from build123d import *

# Parameters (mm, degrees)
F1_DEPTH = 15.24


# Not quite as in the source:
# - a feature names something its author has since deleted; it is built from what else it names


with BuildPart() as f1:
    # F0 (on Top) → F1 (new body)
    with BuildSketch(Plane.XY):
        with BuildLine():
            ThreePointArc((-6.8469626463, 19.8860116913), (-11.313708499, 23.0332541473), (-14.4609509549, 27.5))
            Line((-14.4609509549, 27.5), (-27.5, 14.4609509549))
            Line((-27.5, 14.4609509549), (-21.1890490451, 8.15))
            Line((-21.1890490451, 8.15), (-13.0390490451, 0))
            Line((-13.0390490451, 0), (0, 13.0390490451))
            Line((0, 13.0390490451), (-6.8469626463, 19.8860116913))
        make_face()
        Polygon((-13.0390490451, 0), (-21.1890490451, 8.15), (-21.1890490451, -8.15), align=None)
        with BuildLine():
            Line((14.4609509549, -27.5), (27.5, -14.4609509549))
            Line((27.5, -14.4609509549), (21.1890490451, -8.15))
            Line((21.1890490451, -8.15), (13.0390490451, 0))
            Line((13.0390490451, 0), (0, -13.0390490451))
            Line((0, -13.0390490451), (6.8469626463, -19.8860116913))
            ThreePointArc((6.8469626463, -19.8860116913), (11.313708499, -23.0332541473), (14.4609509549, -27.5))
        make_face()
        Polygon((13.0390490451, 0), (0, 13.0390490451), (0, 0), (0, -13.0390490451), align=None)
        Polygon((0, 0), (0, 13.0390490451), (-13.0390490451, 0), (0, -13.0390490451), align=None)
        with BuildLine():
            Line((27.5, 14.4609509549), (14.4609509549, 27.5))
            ThreePointArc((14.4609509549, 27.5), (11.313708499, 23.0332541473), (6.8469626463, 19.8860116913))
            Line((6.8469626463, 19.8860116913), (0, 13.0390490451))
            Line((0, 13.0390490451), (13.0390490451, 0))
            Line((13.0390490451, 0), (21.1890490451, 8.15))
            Line((21.1890490451, 8.15), (27.5, 14.4609509549))
        make_face()
        Polygon((21.1890490451, -8.15), (21.1890490451, 8.15), (13.0390490451, 0), align=None)
        with BuildLine():
            Line((0, -13.0390490451), (-6.8469626463, -19.8860116913))
            ThreePointArc((-6.8469626463, -19.8860116913), (-3.5089018739, -18.7364659329), (0, -18.3469626463))
            Line((0, -18.3469626463), (0, -13.0390490451))
        make_face()
        with BuildLine():
            Line((0, 13.0390490451), (6.8469626463, 19.8860116913))
            ThreePointArc((6.8469626463, 19.8860116913), (3.5089018739, 18.7364659329), (0, 18.3469626463))
            Line((0, 18.3469626463), (0, 13.0390490451))
        make_face()
        with BuildLine():
            ThreePointArc((0, 18.3469626463), (-3.5089018739, 18.7364659329), (-6.8469626463, 19.8860116913))
            Line((-6.8469626463, 19.8860116913), (0, 13.0390490451))
            Line((0, 13.0390490451), (0, 18.3469626463))
        make_face()
        with BuildLine():
            Line((6.8469626463, -19.8860116913), (0, -13.0390490451))
            Line((0, -13.0390490451), (0, -18.3469626463))
            ThreePointArc((0, -18.3469626463), (3.5089018739, -18.7364659329), (6.8469626463, -19.8860116913))
        make_face()
        with BuildLine():
            Line((-21.1890490451, -8.15), (-27.5, -14.4609509549))
            Line((-27.5, -14.4609509549), (-14.4609509549, -27.5))
            ThreePointArc((-14.4609509549, -27.5), (-11.313708499, -23.0332541473), (-6.8469626463, -19.8860116913))
            Line((-6.8469626463, -19.8860116913), (0, -13.0390490451))
            Line((0, -13.0390490451), (-13.0390490451, 0))
            Line((-13.0390490451, 0), (-21.1890490451, -8.15))
        make_face()
    extrude(amount=F1_DEPTH)


solid = f1.part
Check sheet for the modelled part. Datum: model origin and axes. Units: mm. A direction names the side the tool comes from. Round coordinates to 2 decimals unless told otherwise and drop trailing zeros. Loops run counter-clockwise (first coordinate to the right, second up) from the corner with the lowest first, then second, coordinate; pieces in that order, holes last.
1. Sectioned sample at B-B on z = 8. Record the boundary of the cut face in (x, y), and give its area (3 significant figures).
2. Scan lines: probe 1 along X at (y, z) = (-7, 10.25); probe 2 along X at (y, z) = (-23.5, 9.25); probe 3 along Y at (x, z) = (22.5, 8). Record each from-to range of solid material in increasing order.
3. Sectioned sample at D-D on x = 10. Record the boundary of the cut face in (y, z).
4. Sectioned sample at A-A on x = 22.5. Record the boundary of the cut face in (y, z).
5. Mould release check, pull along Y, two halves, no side actions. Record for faces 1 (the flat face through (24.39, -11.35, 7.51)), 2 (the flat face through (20.89, -21.07, 7.51)), 3 (the flat face through (-24.39, 11.35, 7.51)), 4 (the flat face through (21.07, 20.89, 7.51)): released by +Y, released by -Y, zero draft, split by the parting line, or undercut.
6. Gauge pin test, flat ends, axial feed: pin 1 Ø5 at (y, z) = (-10, 6.5) entering from +X; pin 2 Ø5 at (y, z) = (8.5, 12) entering from -X; pin 3 Ø8 at (y, z) = (-7, 5) entering from +X; pin 4 Ø6 at (x, z) = (15.5, 9.5) entering from -Y. Record the tip position at first contact, or that the pin passes through.
7. Sectioned sample at C-C on y = -4.5. Record the boundary of the cut face in (x, z), and give its area (3 significant figures).
8. Set-up check for faces 5 (the flat face through (21.189, 0, 8)), 6 (the flat face through (-21.07, -20.89, 7.51)), 7 (the flat face through (-24.3, -11.26, 7.51)): record each of +Z, -Z, +X, -X, +Y, -Y from which the full face is reachable in a straight line by a thin tool's end or side.
Recorded:
1. outline: (-27.5, -14.46) - (-14.46, -27.5) arc R16 cw to (14.46, -27.5) - (27.5, -14.46) - (21.19, -8.15) - (21.19, 8.15) - (27.5, 14.46) - (14.46, 27.5) arc R16 cw to (-14.46, 27.5) - (-27.5, 14.46) - (-21.19, 8.15) - (-21.19, -8.15) - close
1. area: 2,020 mm2
2. probe 1: x = -21.19 to 21.19
2. probe 2: x = -18.46 to -11.76, 11.76 to 18.46
2. probe 3: y = -19.46 to -9.46, 9.46 to 19.46
3. outline: (-21.86, 0) - (21.86, 0) - (21.86, 15.24) - (-21.86, 15.24) - close
4. outline: (-19.46, 0) - (-9.46, 0) - (-9.46, 15.24) - (-19.46, 15.24) - close; (9.46, 0) - (19.46, 0) - (19.46, 15.24) - (9.46, 15.24) - close
5. face 1: undercut
5. face 2: released by -Y
5. face 3: undercut
5. face 4: released by +Y
6. pin 1: stops at x = 25.54
6. pin 2: stops at x = -24.04
6. pin 3: stops at x = 24.04
6. pin 4: stops at y = -27.5
7. outline: (-21.19, 0) - (21.19, 0) - (21.19, 15.24) - (-21.19, 15.24) - close
7. area: 646 mm2
8. face 5: +Z, -Z, +X
8. face 6: +Z, -Z, -X, -Y
8. face 7: +Z, -Z, -X
